Could you check a few things on this model? Use its own coordinates, in mm. A direction names the side the tool comes from. Round coordinates to 2 decimals unless told otherwise and drop trailing zeros. Loops run counter-clockwise (first coordinate to the right, second up) from the corner with the lowest first, then second, coordinate; pieces in that order, holes last. Notation, with made-up numbers: (44.5, 16) -> (89.5, 16) arc R14 cw to (89.5, 31) -> close; hole circle Ø5 at (64.25, 52.25). An arc over 180 degrees is marked (long way). Put each result on its own line as item: value. Start each with the question number.
1. Imagine slicing it at D-D, the plane y = -3.5. Please give me the cut outline in (x, z).
2. Imagine slicing it at B-B, the plane y = -13.5. Please give me the cut outline in (x, z) (1 decimal).
3. If we mould it in two halves opening along X, with no side actions, what happens to faces 1 (the flat face through (-9, -17.78, -7)), 2 (the cylindrical face through (10.6, -11.34, 3.34)), 3 (the cylindrical face through (-14.274, -11.341, 0.628))? For each: pulls with the +X half, pulls with the -X half, needs draft (parallel to the pull), parting line crosses it, or undercut.
4. Which directions (+Z, -Z, +X, -X, +Y, -Y) give clear straight access to the entire face, cutting with the end or side of a thin tool? Please do faces 4 (the flat face through (0, 0, 0)), 5 (the flat face through (0, -5.08, 0)).
5. I need wall thicknesses on line 1 (Z direction, x = 0, y = -12.5); line 2 (Y direction, x = 2.75, z = 7); line 3 (X direction, y = -8.75, z = -4.75). Which ranges of each line are inside material? Lowest first, please. Write a range as [from, to].
6. Imagine slicing it at A-A, the plane z = 0. Please give me the cut outline in (x, y).
7. I'm going to push flat-ended pins straight in: P1, Ø1.5, axis at x = 7.5, z = -0.5, coming from the -Y side; P2, Ø5, axis at y = -9.5, z = -11.5, coming from the +X side; P3, Ø10, axis at x = -11, y = -12, coming from the -Z side. Where does each tip first touch, or does it pass through?
8. Imagine slicing it at C-C, the plane x = 0. Please give me the cut outline in (y, z), and give its area (3 significant figures).
```python
from build123d import *

# Parameters (mm, degrees)
F0_R        = 14.2875
F0_R_2      = 11.1125
F1_DEPTH    = 12.7
F1_FACE_R   = 14.2875
F1_FACE_R_2 = 11.1125
F2_DEPTH    = 5.08
F3_R        = 5.08


with BuildPart() as f1:
    # F0 (on Front) → F1 (new body)
    with BuildSketch(Plane.XZ):
        Circle(F0_R)
        Circle(F0_R_2, mode=Mode.SUBTRACT)
    extrude(amount=F1_DEPTH)

    # F0 (on Front) + F1_face (on face) → F2 (join)
    with BuildSketch(Plane.XZ):
        Circle(F0_R_2)
    with BuildSketch(Plane.XZ.offset(12.7)):
        Circle(F1_FACE_R)
        Circle(F1_FACE_R_2, mode=Mode.SUBTRACT)
    extrude(amount=F2_DEPTH)

    # F3
    f3_edges = [f1.edges().sort_by_distance(p)[0] for p in [
        (-14.2875, 0, 0),
    ]]
    fillet(f3_edges, radius=F3_R)


solid = f1.part
```
Entries:
1. outline: circle Ø28.07 at (0, 0)
2. outline: circle Ø28.6 at (0, 0); hole circle Ø22.2 at (0, 0)
3. face 1: needs draft
3. face 2: undercut
3. face 3: parting line crosses it
4. face 4: +Z, -Z, +X, -X, +Y
4. face 5: -Y
5. line 1: [-14.29, -11.11], [11.11, 14.29]
5. line 2: [-5.08, 0]
5. line 3: [-13.47, -10.05], [10.05, 13.47]
6. outline: (-14.29, -17.78) -> (-11.11, -17.78) -> (-11.11, -5.08) -> (11.11, -5.08) -> (11.11, -17.78) -> (14.29, -17.78) -> (14.29, -5.08) arc R5.08 ccw to (9.21, 0) -> (-9.21, 0) arc R5.08 ccw to (-14.29, -5.08) -> close
7. P1: y = -5.08
7. P2: x = 11.1
7. P3: z = -12.97
8. outline: (-17.78, -14.29) -> (-5.08, -14.29) arc R5.08 ccw to (0, -9.21) -> (0, 9.21) arc R5.08 ccw to (-5.08, 14.29) -> (-17.78, 14.29) -> (-17.78, 11.11) -> (-5.08, 11.11) -> (-5.08, -11.11) -> (-17.78, -11.11) -> close
8. area: 215 mm^2
